Build history of the part. All positions in model axes, mm. Face numbers are marked on the shaded views. Give positions to 0.01 mm unless a question says otherwise; leave off trailing zeros. Write each loop counter-clockwise with the first axis right and the second up, starting at its lowest first coordinate (ties: lowest second). Pieces come first, ordered by that corner, then holes. Notation, with made-up numbers: M 11.25,0.5 L 61.25,0.5 A22 ccw 61.25,34.5 Z; hole C -14,69 d1. An arc over 180 degrees is marked long. One line per item, written item: value. Start each with the question number.
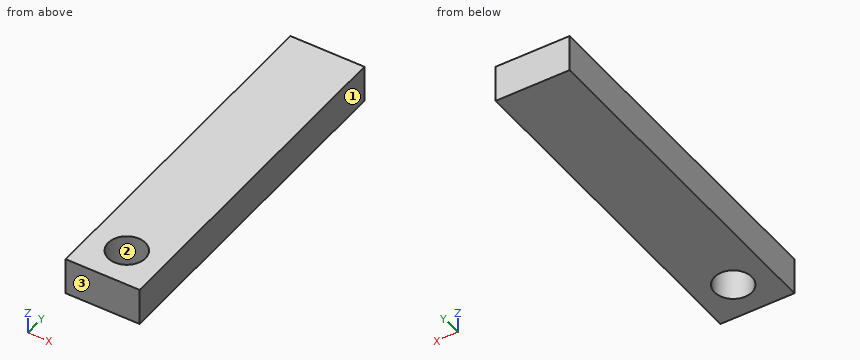
Autodesk Inventor part; units mm, degrees
ref_plane "YZ Plane" through (0, 0, 0) normal (1, 0, 0) x (0, 1, 0)
ref_plane "XZ Plane" through (0, 0, 0) normal (0, 1, 0) x (-1, 0, 0)
ref_plane "XY Plane" through (0, 0, 0) normal (0, 0, 1) x (1, 0, 0)
sketch "Sketch2" plane through (0, 0, 0) normal (0, 0, 1) x (1, 0, 0)
  line L0 (0, 0) -> (-9.9, 0)
  line L1 (-4.95, 0) -> (-4.95, 2.5)
  line L2 (-4.95, 0) -> (-2.45, 0) construction
  circle A0 centre (-4.95, 5) radius 2.5
  line L3 (-4.95, 7.5) -> (32.05, 7.5) construction
  line L4 (0, 44.5) -> (0, 0)
  line L5 (0, 0) -> (-9.9, 0)
  line L6 (-9.9, 0) -> (-9.9, 44.5)
  line L7 (0, 45.5) -> (0, 0)
  line L8 (0, 0) -> (-9.9, 0)
  line L9 (-9.9, 0) -> (-9.9, 45.5)
  line L10 (-4.95, 7.5) -> (66.05, 7.5) construction
  line L11 (0, 0) -> (-9.9, 0)
  line L12 (-9.9, 0) -> (-9.9, 46.5)
  line L13 (-9.9, 46.5) -> (0, 46.5)
  line L14 (0, 46.5) -> (0, 0)
  dimension "d35" = 5
  dimension "d33" = 2.5
  dimension "d34" = 90
  dimension "d46" = 46.5
extrude "Extrusion6" add sketch "Sketch2" along normal blind 5
properties part number "Elbow_Cube_Holder_TestFit_V2"
1) Mould opens along X. For the marked faces 1, 2 and 3 say: released by +X, released by -X, zero draft, split by the parting line, or undercut.
2) Drop flat-ended pins along their axis: P1, Ø1.5, axis at x = -2.5, y = 26.5, coming from the -Z side; P2, Ø4, axis at x = -4.95, y = 5, coming from the -Z side. Give the stop position or say it passes through.
3) Band-saw the part on B-B (y = 5). List the corners of the cut face in (x, z), then the cut area to 3 significant figures.
4) Band-saw the part on A-A (x = -4.95). List the corners of the cut face in (y, z), then the cut area to 4 significant figures.
5) Probe line 1 along Y through (x, z) = (-4.95, 1.6); line 2 along X through (y, z) = (5, 3.4); line 3 along Y through (x, z) = (-5.5, 3.65). List the from-to ranges inside material, lowest first. Write a range as from..to.
6) Band-saw the part on C-C (z = 3.05). List the corners of the cut face in (x, y), then the cut area to 3 significant figures.
Model answer:
1. face 1: released by +X
1. face 2: undercut
1. face 3: zero draft
2. P1: stops at z = 0
2. P2: passes through
3. outline: M -9.9,0 L -7.45,0 L -7.45,5 L -9.9,5 Z; M -2.45,0 L 0,0 L 0,5 L -2.45,5 Z
3. area: 24.5 mm²
4. outline: M 0,0 L 2.5,0 L 2.5,5 L 0,5 Z; M 7.5,0 L 46.5,0 L 46.5,5 L 7.5,5 Z
4. area: 207.5 mm²
5. line 1: y = 0..2.5, 7.5..46.5
5. line 2: x = -9.9..-7.45, -2.45..0
5. line 3: y = 0..2.56, 7.44..46.5
6. outline: M -9.9,0 L 0,0 L 0,46.5 L -9.9,46.5 Z; hole C -4.95,5 d5
6. area: 441 mm²
